```python
from build123d import *

# Parameters (mm, degrees)
SKETCH_1_R          = 7.5
EXTRUDE_1_DEPTH     = 5
SKETCH_2_W          = 2
SKETCH_2_H          = 2
EXTRUDE_2_DEPTH     = 7
SKETCH_3_R          = 10
EXTRUDE_3_DEPTH     = 40
CUT_EXTRUDE_1_DEPTH = 2


with BuildPart() as part:
    # 草图1 → 凸台-拉伸1 (new body)
    with BuildSketch(Plane.XY):
        Circle(SKETCH_1_R)
    extrude(amount=EXTRUDE_1_DEPTH)

    # 草图2 → 凸台-拉伸2 (add)
    with BuildSketch(Plane(origin=(0, 0, 0), x_dir=(-1, 0, 0), z_dir=(0, 0, -1))):
        with Locations((-2, 0)):
            Rectangle(SKETCH_2_W, SKETCH_2_H)
        with Locations((0, 2)):
            Rectangle(SKETCH_2_W, SKETCH_2_H)
        with Locations((2, 0)):
            Rectangle(SKETCH_2_W, SKETCH_2_H)
        Rectangle(SKETCH_2_W, SKETCH_2_H)
        with Locations((0, -2)):
            Rectangle(SKETCH_2_W, SKETCH_2_H)
    extrude(amount=EXTRUDE_2_DEPTH)

    # 草图3 → 凸台-拉伸3 (add)
    with BuildSketch(Plane.XY.offset(5)):
        Circle(SKETCH_3_R)
    extrude(amount=EXTRUDE_3_DEPTH)

    # 草图4 → 切除-拉伸1 (cut)
    with BuildSketch(Plane(origin=(0, 10, 0), x_dir=(1, 0, 0), z_dir=(0, 1, 0))):
        with BuildLine():
            Line((-2, -41), (-2, -33))
            ThreePointArc((-2, -33), (0, -31), (2, -33))
            Line((2, -33), (2, -41))
            ThreePointArc((2, -41), (0, -43), (-2, -41))
        make_face()
    extrude(amount=-CUT_EXTRUDE_1_DEPTH, mode=Mode.SUBTRACT)


solid = part.part
```
The model under review builds one solid part; all positions refer to its coordinate system, in mm. A direction names the side the tool comes from. Coordinates: 2 decimals unless noted, no trailing zeros. Order: outer loops, then holes, each group sorted by start corner. A loop starts at its lowest first (then second) coordinate and runs counter-clockwise, first axis right, second up. Notation, with made-up numbers: M 1.25,15 L 59.25,15 A14 ccw 59.25,23 Z; hole C 50.5,14 d1. An arc over 180 degrees is marked long. One line per question, with ' | ' between items.
(1) Machinability: for faces 1 (the face through (0, 9, 31)), 2 (the face through (2, 1, -3)), 3 (the face through (-1, 2, -3)), 4 (the face through (3, 0, -3)), which of the approach directions +Z, -Z, +X, -X, +Y, -Y give a long, thin tool a straight path to every point of the face, cutting with its end or side? Answer none if there is none.
Geometry results:
face 1: +Y | face 2: -Z, +X, +Y | face 3: -Z, -X, +Y | face 4: -Z, +X, +Y, -Y
(2) Insertion check: pin 1 (3 mm diameter, centred on y = 5.5, z = 4, fed in from -X); pin 2 (1.6 mm diameter, centred on x = 2, z = -3, fed in from +Y); pin 3 (1.5 mm diameter, centred on x = -6.5, y = 3.5, fed in from -Z). Each pin has a flat end and moves straight along its axis. Give the tip position at first contact, or say it passes through.
Geometry results:
pin 1: stops at x = -8.99 | pin 2: stops at y = 1 | pin 3: stops at z = 0
(3) Add section D-D, the plane y = 2.25. Write out the cut boundary in (x, z).
Geometry results:
outline: M -9.74,5 L -7.15,5 L -7.15,0 L -1,0 L -1,-7 L 1,-7 L 1,0 L 7.15,0 L 7.15,5 L 9.74,5 L 9.74,45 L -9.74,45 Z
(4) Add section A-A, the plane x = 0. Write out the cut boundary in (y, z).
Geometry results:
outline: M -10,5 L -7.5,5 L -7.5,0 L -3,0 L -3,-7 L 3,-7 L 3,0 L 7.5,0 L 7.5,5 L 10,5 L 10,31 L 8,31 L 8,43 L 10,43 L 10,45 L -10,45 Z
(5) Add section C-C, the plane z = 1.5. Write out the cut boundary in (x, y), then the cut area to 3 significant figures.
Geometry results:
outline: C 0,0 d15 | area: 177 mm²
(6) The part is to be moulded in two halves that separate along Z. For faces 5 (the face through (-1, -2, -3)), 6 (the face through (2, 9, 37)), 7 (the face through (0, 0, 45)), say which applies: +Z half, -Z half, draft (parallel to the pull), parting line (faces both ways), or undercut.
Geometry results:
face 5: draft | face 6: undercut | face 7: +Z half
(7) For probe 1 along Z at (x, y) = (0.75, -4.75); probe 2 along Z at (x, y) = (2.25, 9.25); probe 3 along X at (y, z) = (6.5, 3.5), list the stretches that pass through material, from the lowest coordinate up. Write a range as from..to.
Geometry results:
probe 1: z = 0..45 | probe 2: z = 5..45 | probe 3: x = -3.74..3.74
(8) Add section B-B, the plane y = 0. Write out the cut boundary in (x, z).
Geometry results:
outline: M -10,5 L -7.5,5 L -7.5,0 L -3,0 L -3,-7 L 3,-7 L 3,0 L 7.5,0 L 7.5,5 L 10,5 L 10,45 L -10,45 Z
